from build123d import *

# Parameters (mm, degrees)
SKETCH1_R           = 30
SKETCH1_R_2         = 15
BOSS_EXTRUDE1_DEPTH = 25
BOSS_EXTRUDE2_DEPTH = 5


with BuildPart() as part:
    # Sketch1 → Boss-Extrude1 (new body, symmetric)
    with BuildSketch(Plane(origin=(0, 0, 0), x_dir=(1, 0, 0), z_dir=(0, 1, 0))):
        with Locations(Location((0, 0, 0), (0, 0, 270))):  # turned: the seam where the file's is
            Circle(SKETCH1_R)
        with Locations(Location((0, 0, 0), (0, 0, 270))):  # turned: the seam where the file's is
            Circle(SKETCH1_R_2, mode=Mode.SUBTRACT)
    extrude(amount=BOSS_EXTRUDE1_DEPTH, both=True)

    # Sketch2 → Boss-Extrude2 (add, symmetric)
    with BuildSketch(Plane(origin=(0, 0, 0), x_dir=(1, 0, 0), z_dir=(0, 1, 0))):
        with BuildLine():
            Line((-122.5, 15), (-122.5, -15))
            Line((-122.5, -15), (-97.5, -15))
            Line((-97.5, -15), (-4.671688756, -29.634023084))
            ThreePointArc((-4.671688756, -29.634023084), (-30, 0), (-4.671688756, 29.634023084))
            Line((-4.671688756, 29.634023084), (-97.5, 15))
            Line((-97.5, 15), (-122.5, 15))
        make_face()
    extrude(amount=BOSS_EXTRUDE2_DEPTH, both=True)


solid = part.part
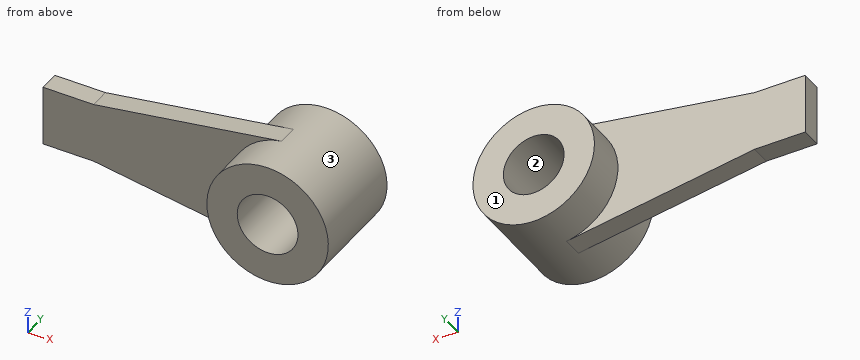
CAD build for the part. Positions are in the model's coordinates, mm. Face numbers are marked on the shaded views. Give positions to 0.01 mm unless a question says otherwise; leave off trailing zeros. Order: outer loops, then holes, each group sorted by start corner. A loop starts at its lowest first (then second) coordinate and runs counter-clockwise, first axis right, second up. Notation, with made-up numbers: (10.5, -20) - (65.5, -20) arc R5 ccw to (65.5, -13) - close; hole circle Ø5 at (-5.75, -1). An arc over 180 degrees is marked (long way). Answer in a Markdown table with one row per item.
1. Flat gauge pins, fed straight in: pin 1 (12 mm diameter, centred on x = 13.5, y = -7, fed in from +Z); pin 2 (5 mm diameter, centred on x = -106, y = -1.5, fed in from +Z); pin 3 (5 mm diameter, centred on x = -35.5, z = -19, fed in from +Y). Where does each tip first touch, or does it go through?
Data:
| item | result |
|---|---|
| pin 1 | stops at z = 29.05 |
| pin 2 | stops at z = 15 |
| pin 3 | stops at y = 5 |
2. Saw through at D-D, the plane z = 24. Give the cut face in (x, y), plus the area to 3 significant figures.
Data:
| item | result |
|---|---|
| outline | (-40.41, -5) - (-18, -5) - (-18, -25) - (18, -25) - (18, 25) - (-18, 25) - (-18, 5) - (-40.41, 5) - close |
| area | 2,020 mm² |
3. Saw through at B-B, the plane y = 0. Give the cut face in (x, z), plus the area to 3 significant figures.
Data:
| item | result |
|---|---|
| outline | (-122.5, -15) - (-97.5, -15) - (-4.67, -29.63) arc R30 ccw (long way) to (-4.67, 29.63) - (-97.5, 15) - (-122.5, 15) - close; hole circle Ø30 at (0, 0) |
| area | 5,880 mm² |
4. Saw through at C-C, the plane z = 0. Give the cut face in (x, y), plus the area to 4 significant figures.
Data:
| item | result |
|---|---|
| outline | (-122.5, -5) - (-30, -5) - (-30, -25) - (-15, -25) - (-15, 25) - (-30, 25) - (-30, 5) - (-122.5, 5) - close; (15, -25) - (30, -25) - (30, 25) - (15, 25) - close |
| area | 2,425 mm² |
5. Pull direction Z, two halves, no side cores. Call the marked faces 1, 2 and 3: pulls with the +Z half, pulls with the -Z half, needs draft (parallel to the pull), parting line crosses it, or undercut.
Data:
| item | result |
|---|---|
| face 1 | needs draft |
| face 2 | undercut |
| face 3 | parting line crosses it |
6. Saw through at A-A, the plane x = 0. Give the cut face in (y, z).
Data:
| item | result |
|---|---|
| outline | (-25, -30) - (25, -30) - (25, -15) - (-25, -15) - close; (-25, 15) - (25, 15) - (25, 30) - (-25, 30) - close |
7. Probe probe 1 along X at (y, z) = (-19, 0.5); probe 2 along X at (y, z) = (1, 0); probe 3 along Y at (x, z) = (-73, -12.5). List the from-to ranges inside material, lowest first. Write a range as [from, to].
Data:
| item | result |
|---|---|
| probe 1 | x = [-30, -14.99], [14.99, 30] |
| probe 2 | x = [-122.5, -15], [15, 30] |
| probe 3 | y = [-5, 5] |
